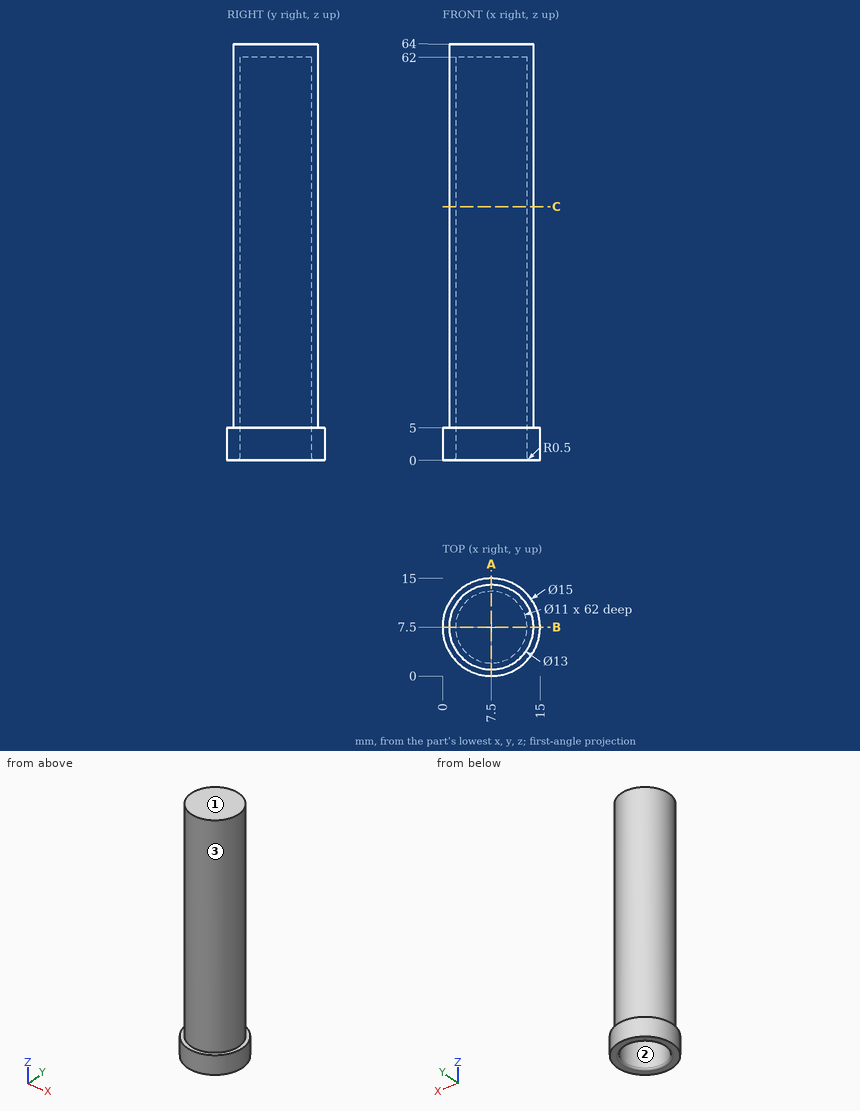
Geometry: see drawing. Coordinates: mm, zero at the bounding-box minimum. Give positions to 0.01 mm unless a question says otherwise; leave off trailing zeros. Write each loop counter-clockwise with the first axis right and the second up, starting at its lowest first coordinate (ties: lowest second). Pieces come first, ordered by that corner, then holes. Notation, with made-up numbers: (39, 85) - (75, 85) arc R33 ccw to (75, 116) - close; hole circle Ø9 at (-27, 67). An arc over 180 degrees is marked (long way). Return JSON: item names as keys, results as strings. Group by question number.
1) First-contact query: P1, Ø4, axis at x = 6, y = 11, coming from the -Z side; P2, Ø8, axis at x = 2, z = 42.5, coming from the +Y side; P3, Ø6.5, axis at x = 7.5, y = 7.5, coming from the -Z side. Flat tips, straight axial feed; report the tip coordinate or a pass-through.
2) Section C-C on z = 39. Return the cut outline in (x, y), plus the area to 3 significant figures.
3) Line query: line 1 (Y direction, x = 7.5, z = 28); line 2 (Y direction, x = 8.5, z = 43); line 3 (X direction, y = 7, z = 35). Output: solid intervals per line, ascending.
4) Mould query, pull axis X, two halves, no side actions, for the marked faces 1, 2 and 3. Classes: released by +X, released by -X, zero draft, split by the parting line, or undercut.
5) Section A-A on x = 7.5. Return the cut outline in (y, z).
Filled in:
{
 "1": {"P1": "stops at z = 0.04", "P2": "stops at y = 13.82", "P3": "stops at z = 62"},
 "2": {"outline": "circle Ø13 at (7.5, 7.5); hole circle Ø11 at (7.5, 7.5)", "area": "37.7 mm^2"},
 "3": {"line 1": "y = 1 to 2, 13 to 14", "line 2": "y = 1.08 to 2.09, 12.91 to 13.92", "line 3": "x = 1.02 to 2.02, 12.98 to 13.98"},
 "4": {"face 1": "zero draft", "face 2": "undercut", "face 3": "split by the parting line"},
 "5": {"outline": "(0, 0) - (1.5, 0) arc R0.5 ccw to (2, 0.5) - (2, 62) - (13, 62) - (13, 0.5) arc R0.5 ccw to (13.5, 0) - (15, 0) - (15, 5) - (14, 5) - (14, 64) - (1, 64) - (1, 5) - (0, 5) - close"}
}
